Build history of the part. All positions in model axes, mm. Face numbers are marked on the shaded views. A direction names the side the tool comes from. Round coordinates to 2 decimals unless told otherwise and drop trailing zeros. Loops run counter-clockwise (first coordinate to the right, second up) from the corner with the lowest first, then second, coordinate; pieces in that order, holes last. Notation, with made-up numbers: (68, 52) - (119, 52) arc R21 ccw to (119, 91) - close; hole circle Ø6 at (15, 79.25). An arc over 180 degrees is marked (long way). Use a Markdown table: item, result.
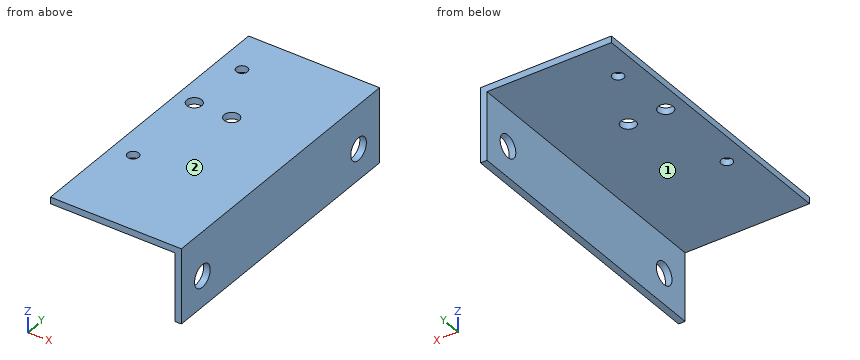
from build123d import *

# Parameters (mm, degrees)
BOSS_EXTRUDE1_DEPTH = 76
CUT_EXTRUDE1_REACH  = 3.75
SKETCH3_R           = 3
CUT_EXTRUDE2_REACH  = 22
SKETCH4_R           = 1.5
SKETCH4_R_2         = 2


with BuildPart() as part:
    # Sketch1 → Boss-Extrude1 (new body)
    with BuildSketch(Plane(origin=(0, 0, 0), x_dir=(1, 0, 0), z_dir=(0, 1, 0))):
        Polygon((-35, 0), (-35, -1.75), (0, -1.75), (0, 18.25), (-1.75, 18.25), (-1.75, 0), align=None)
    extrude(amount=BOSS_EXTRUDE1_DEPTH)

    # Sketch3 → Cut-Extrude1 (cut, up to next)
    with BuildSketch(Plane.ZY.offset(1.75), mode=Mode.PRIVATE) as cut_extrude1_sk1:
        with Locations((-10, 8.05)):
            Circle(SKETCH3_R)
    cut_extrude1_tool1 = extrude(cut_extrude1_sk1.sketch, amount=-CUT_EXTRUDE1_REACH, mode=Mode.PRIVATE) & part.part
    add(cut_extrude1_tool1.solids().sort_by_distance((-1.75, 8.05, -10))[0], mode=Mode.SUBTRACT)
    # Sketch3 → Cut-Extrude1 (cut, up to next)
    with BuildSketch(Plane.ZY.offset(1.75), mode=Mode.PRIVATE) as cut_extrude1_sk2:
        with Locations((-10, 67.955)):
            Circle(SKETCH3_R)
    cut_extrude1_tool2 = extrude(cut_extrude1_sk2.sketch, amount=-CUT_EXTRUDE1_REACH, mode=Mode.PRIVATE) & part.part
    add(cut_extrude1_tool2.solids().sort_by_distance((-1.75, 67.955, -10))[0], mode=Mode.SUBTRACT)

    # Sketch4 → Cut-Extrude2 (cut, up to next)
    with BuildSketch(Plane.XY.offset(1.75), mode=Mode.PRIVATE) as cut_extrude2_sk1:
        with Locations((-28.76701924, 64.5)):
            Circle(SKETCH4_R)
    cut_extrude2_tool1 = extrude(cut_extrude2_sk1.sketch, amount=-CUT_EXTRUDE2_REACH, mode=Mode.PRIVATE) & part.part
    add(cut_extrude2_tool1.solids().sort_by_distance((-28.767019, 64.5, 1.75))[0], mode=Mode.SUBTRACT)
    # Sketch4 → Cut-Extrude2 (cut, up to next)
    with BuildSketch(Plane.XY.offset(1.75), mode=Mode.PRIVATE) as cut_extrude2_sk2:
        with Locations((-29.41701924, 23.7)):
            Circle(SKETCH4_R)
    cut_extrude2_tool2 = extrude(cut_extrude2_sk2.sketch, amount=-CUT_EXTRUDE2_REACH, mode=Mode.PRIVATE) & part.part
    add(cut_extrude2_tool2.solids().sort_by_distance((-29.417019, 23.7, 1.75))[0], mode=Mode.SUBTRACT)
    # Sketch4 → Cut-Extrude2 (cut, up to next)
    with BuildSketch(Plane.XY.offset(1.75), mode=Mode.PRIVATE) as cut_extrude2_sk3:
        with Locations((-30, 48)):
            Circle(SKETCH4_R_2)
    cut_extrude2_tool3 = extrude(cut_extrude2_sk3.sketch, amount=-CUT_EXTRUDE2_REACH, mode=Mode.PRIVATE) & part.part
    add(cut_extrude2_tool3.solids().sort_by_distance((-30, 48, 1.75))[0], mode=Mode.SUBTRACT)
    # Sketch4 → Cut-Extrude2 (cut, up to next)
    with BuildSketch(Plane.XY.offset(1.75), mode=Mode.PRIVATE) as cut_extrude2_sk4:
        with Locations((-20, 48)):
            Circle(SKETCH4_R_2)
    cut_extrude2_tool4 = extrude(cut_extrude2_sk4.sketch, amount=-CUT_EXTRUDE2_REACH, mode=Mode.PRIVATE) & part.part
    add(cut_extrude2_tool4.solids().sort_by_distance((-20, 48, 1.75))[0], mode=Mode.SUBTRACT)


solid = part.part
Q1. Cut at A-A, the plane y = 23.7. List the corners of the cut face in (x, z), plus the area to 3 significant figures.
Results found:
| item | result |
|---|---|
| outline | (-35, 0) - (-30.92, 0) - (-30.92, 1.75) - (-35, 1.75) - close; (-27.92, 0) - (-1.75, 0) - (-1.75, -18.25) - (0, -18.25) - (0, 1.75) - (-27.92, 1.75) - close |
| area | 87.9 mm2 |
Q2. Probe line 1 (Y direction, x = -1.35, z = -10) (3 decimals); line 2 (X direction, y = 50, z = -5.75); line 3 (Z direction, x = -9.5, y = 54.5). List the from-to ranges inside material, lowest first.
Results found:
| item | result |
|---|---|
| line 1 | y = 0 to 5.05, 11.05 to 64.955, 70.955 to 76 |
| line 2 | x = -1.75 to 0 |
| line 3 | z = 0 to 1.75 |
Q3. Cut at B-B, the plane z = -10. List the corners of the cut face in (x, y) (3 decimals), plus the area to 3 significant figures.
Results found:
| item | result |
|---|---|
| outline | (-1.75, 0) - (0, 0) - (0, 5.05) - (-1.75, 5.05) - close; (-1.75, 11.05) - (0, 11.05) - (0, 64.955) - (-1.75, 64.955) - close; (-1.75, 70.955) - (0, 70.955) - (0, 76) - (-1.75, 76) - close |
| area | 112 mm2 |
Q4. Cut at D-D, the plane y = 8.05. List the corners of the cut face in (x, z).
Results found:
| item | result |
|---|---|
| outline | (-35, 0) - (-1.75, 0) - (-1.75, -7) - (0, -7) - (0, 1.75) - (-35, 1.75) - close; (-1.75, -18.25) - (0, -18.25) - (0, -13) - (-1.75, -13) - close |
Q5. Which spindle directions (+Z, -Z, +X, -X, +Y, -Y) get a long thin tool onto all of the face, cutting with end or side? Do the marked faces 1 and 2. Say none if no direction does.
Results found:
| item | result |
|---|---|
| face 1 | -Z, -X, +Y, -Y |
| face 2 | +Z, +X, -X, +Y, -Y |
Q6. Cut at C-C, the plane x = -20. List the corners of the cut face in (y, z), plus the area to 3 significant figures.
Results found:
| item | result |
|---|---|
| outline | (0, 0) - (46, 0) - (46, 1.75) - (0, 1.75) - close; (50, 0) - (76, 0) - (76, 1.75) - (50, 1.75) - close |
| area | 126 mm2 |
Q7. Drop flat-ended pins along their axis: pin 1 (4 mm diameter, centred on y = 13.5, z = -3.5, fed in from +X); pin 2 (8 mm diameter, centred on x = -31, y = 47.5, fed in from -Z); pin 3 (3.5 mm diameter, centred on x = -20, y = 48, fed in from +Z); pin 4 (9.5 mm diameter, centred on y = 67.955, z = -10, fed in from -X). Give the stop position or say it passes through.
Results found:
| item | result |
|---|---|
| pin 1 | stops at x = 0 |
| pin 2 | stops at z = 0 |
| pin 3 | passes through |
| pin 4 | stops at x = -1.75 |
